from build123d import *

# Parameters (mm, degrees)
F1_DEPTH = 10.16
F2_R     = 6.985
F3_DEPTH = 6.35
F4_R     = 7.62


with BuildPart() as f1:
    # F0 (on Top) → F1 (new body)
    with BuildSketch(Plane.XY):
        Polygon((21.997045, 12.7), (-21.997045, 12.7), (0, -25.4), align=None)
        Polygon((-11.071846, 0), (-5.535923, 9.5885), (5.535923, 9.5885), (11.071846, 0), (5.535923, -9.5885), (-5.535923, -9.5885), align=None, mode=Mode.SUBTRACT)
    extrude(amount=F1_DEPTH)

    # F2 (on face) → F3 (join)
    with BuildSketch(Plane.XY.offset(10.16)):
        Polygon((21.997045, 12.7), (-21.997045, 12.7), (0, -25.4), align=None)
        Polygon((-5.535923, -9.5885), (-11.071846, 0), (-5.535923, 9.5885), (5.535923, 9.5885), (11.071846, 0), (5.535923, -9.5885), align=None, mode=Mode.SUBTRACT)
        Polygon((-5.535923, 9.5885), (-11.071846, 0), (-5.535923, -9.5885), (5.535923, -9.5885), (11.071846, 0), (5.535923, 9.5885), align=None)
        Circle(F2_R, mode=Mode.SUBTRACT)
    extrude(amount=F3_DEPTH)

    # F4
    f4_edges = [f1.edges().sort_by_distance(p)[0] for p in [
        (-21.997045, 12.7, 8.255),
        (21.997045, 12.7, 8.255),
        (0, -25.4, 8.255),
    ]]
    fillet(f4_edges, radius=F4_R)


solid = f1.part
The listing builds one solid part. Answer for the finished solid, in the listing's coordinates (mm). A direction names the side the tool comes from. Round coordinates to 2 decimals unless told otherwise and drop trailing zeros. Order: outer loops, then holes, each group sorted by start corner. A loop starts at its lowest first (then second) coordinate and runs counter-clockwise, first axis right, second up. Notation, with made-up numbers: M -28.5,-29 L 28.5,-29 A32 cw 28.5,6 Z; hole C 33.5,62.25 d3. An arc over 180 degrees is marked long. Answer in a Markdown table with one row per item. Add a question column.
1) Consider line 1 along X through (y, z) = (-1, 10.25); line 2 along X through (y, z) = (4.5, 13.75); line 3 along Y through (x, z) = (3.5, 1.5). Determine where each line is inside the solid, lowest interval first. Write a range as from..to.
2) The part is cut by section A-A on x = 0. Determine the outline of the cut face in (y, z) (1 decimal).
3) Determine the mould class of faces 3 (the face through (7, 8, 0)), 4 (the face through (15.34, 8.99, 8.14)), 5 (the face through (-11.06, -6.24, 8.14)), 6 (the face through (0, 9.588, 5)) for opening direction X: pulls with the +X half, pulls with the -X half, needs draft (parallel to the pull), parting line crosses it, or undercut.
4) Flat-ended cylindrical pins translate along their axes: pin 1 Ø4 at (y, z) = (-5.5, 9) entering from +X; pin 2 Ø8 at (x, z) = (-10, 12) entering from -Y; pin 3 Ø4 at (y, z) = (-2.5, 2.5) entering from +X. Find the tip coordinate at first contact, or state that the pin passes through.
5) The part is cut by section C-C on z = 14.5. Determine the outline of the cut face in (x, y) (3 decimals).
6) The part is cut by section B-B on y = 5. Determine the outline of the cut face in (x, z).
7) Which of the six approach directions +Z, -Z, +X, -X, +Y, -Y give full straight-line access (tool end or side, diameter ignored) to faces 1 (the face through (10.937, -6.457, 8.139)), 2 (the face through (-8.265, -4.861, 5.009))?
Findings below:
| question | item | result |
|---|---|---|
| 1 | line 1 | x = -14.09..-6.91, 6.91..14.09 |
| 1 | line 2 | x = -16.4..-5.34, 5.34..16.4 |
| 1 | line 3 | y = -16.93..-9.59, 9.59..12.7 |
| 2 | outline | M -17.8,0 L -9.6,0 L -9.6,10.2 L -7,10.2 L -7,16.5 L -17.8,16.5 Z; M 7,10.2 L 9.6,10.2 L 9.6,0 L 12.7,0 L 12.7,16.5 L 7,16.5 Z |
| 3 | face 3 | needs draft |
| 3 | face 4 | pulls with the +X half |
| 3 | face 5 | pulls with the -X half |
| 3 | face 6 | undercut |
| 4 | pin 1 | stops at x = 12.64 |
| 4 | pin 2 | stops at y = -14.86 |
| 4 | pin 3 | stops at x = 14.38 |
| 5 | outline | M -15.398,1.27 L -6.599,-13.97 A7.62 ccw 6.599,-13.97 L 15.398,1.27 A7.62 ccw 8.799,12.7 L -8.799,12.7 A7.62 ccw Z; hole C 0,0 d13.97 |
| 6 | outline | M -16.42,0 L -8.19,0 L -8.19,10.16 L -4.88,10.16 L -4.88,16.51 L -16.42,16.51 Z; M 4.88,10.16 L 8.19,10.16 L 8.19,0 L 16.42,0 L 16.42,16.51 L 4.88,16.51 Z |
| 7 | face 1 | +Z, -Z, +X, -Y |
| 7 | face 2 | -Z |
